from build123d import *

# Parameters (mm, degrees)
PAD_DEPTH    = 51.96
PAD001_DEPTH = 26
SKETCH002_R  = 2
POCKET_DEPTH = 45.899584
FILLET_R     = 3


with BuildPart() as part:
    # Sketch → Pad (new body)
    with BuildSketch(Plane.XY):
        with BuildLine():
            Line((-48.25, -23), (-52.123371, -6.118146))
            ThreePointArc((-47.25, 0), (-51.160929, -1.884774), (-52.123371, -6.118146))
            Line((-47.25, 0), (47.25, 0))
            ThreePointArc((52.123371, -6.118146), (51.160929, -1.884774), (47.25, 0))
            Line((52.123371, -6.118146), (48.25, -23))
            Line((48.25, -23), (47.25, -23))
            Line((47.25, -23), (47.25, -8))
            ThreePointArc((47.25, -8), (45.785534, -4.464466), (42.25, -3))
            Line((42.25, -3), (-42.25, -3))
            ThreePointArc((-42.25, -3), (-45.785534, -4.464466), (-47.25, -8))
            Line((-47.25, -8), (-47.25, -23))
            Line((-47.25, -23), (-48.25, -23))
        make_face()
    extrude(amount=PAD_DEPTH)

    # Sketch001 → Pad001 (join, symmetric)
    with BuildSketch(Plane.YZ):
        Polygon((0, 51.96), (29.99912, 51.96), (0, 0), (0, 6), (24.802968, 48.96), (0, 48.96), align=None)
    extrude(amount=PAD001_DEPTH, both=True)

    # Sketch002 (on Face15 of Pad001) → Pocket (cut, through all)
    with BuildSketch(Plane(origin=(0, 0, 0), x_dir=(-1, 0, 0), z_dir=(0, 0.866025, -0.5))):
        with Locations((-18, 49.99824)):
            Circle(SKETCH002_R)
        with Locations((18, 49.99824)):
            Circle(SKETCH002_R)
        with Locations((-18, 27.99824)):
            Circle(SKETCH002_R)
        with Locations((18, 27.99824)):
            Circle(SKETCH002_R)
    extrude(amount=-POCKET_DEPTH, mode=Mode.SUBTRACT)

    # Fillet
    fillet_edges = [part.edges().sort_by_distance(p)[0] for p in [
        (0, 0, 48.96),
        (0, 0, 6),
    ]]
    fillet(fillet_edges, radius=FILLET_R)


solid = part.part
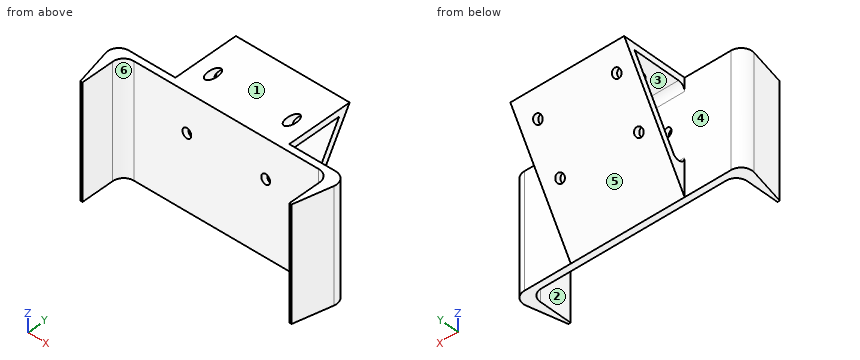
Check sheet for the modelled part. Datum: model origin and axes. Units: mm. Face numbers are marked on the shaded views. A direction names the side the tool comes from. Round coordinates to 2 decimals unless told otherwise and drop trailing zeros. Loops run counter-clockwise (first coordinate to the right, second up) from the corner with the lowest first, then second, coordinate; pieces in that order, holes last. Notation, with made-up numbers: (54, -23.5) - (69, -23.5) arc R26 cw to (69, -8.5) - close; hole circle Ø7 at (1, 10.5). An arc over 180 degrees is marked (long way). Answer as CSV lines item,"result". Start each with the question number.
Item 1: Scan lines: line 1 (Y direction, x = 37, z = 17); line 2 (X direction, y = -10, z = 9); line 3 (X direction, y = 0.5, z = 14.5). Record each from-to range of solid material in increasing order. Write a range as [from, to].
Item 2: Depth check by flat-ended pin: P1, Ø24, axis at y = 14.5, z = 34, coming from the +X side; P2, Ø11, axis at x = 8.5, y = 16.5, coming from the -Z side; P3, Ø12, axis at x = -36, z = 30, coming from the -Y side. Enter the tip coordinate at first touch or a pass-through.
Item 3: Section check B-B (y = -18). Record the boundary of the cut face in (x, z).
Item 4: Release check for a two-part mould opening along Z. For the marked faces 1, 2 and 3 record: +Z half, -Z half, draft (parallel to the pull), parting line (faces both ways), or undercut.
Item 5: Section check A-A (x = -9). Record the boundary of the cut face in (y, z).
Item 6: Set-up check for the marked faces 4, 5 and 6: record each of +Z, -Z, +X, -X, +Y, -Y from which the full face is reachable in a straight line by a thin tool's end or side.
Item 7: Section check C-C (z = 37.5). Record the boundary of the cut face in (x, y), and give its area (3 significant figures).
Item 8: Section check D-D (x = -37). Record the boundary of the cut face in (y, z), and give its area (3 significant figures).
Report:
1,line 1,"y = [-3, 0]"
1,line 2,"x = [-51.23, -47.25], [47.25, 51.23]"
1,line 3,"x = [-26, 26]"
2,P1,"stops at x = 26"
2,P2,"stops at z = 19.05"
2,P3,"stops at y = -3"
3,outline,"(-49.4, 0) - (-47.25, 0) - (-47.25, 51.96) - (-49.4, 51.96) - close; (47.25, 0) - (49.4, 0) - (49.4, 51.96) - (47.25, 51.96) - close"
4,face 1,"+Z half"
4,face 2,"draft"
4,face 3,"undercut"
5,outline,"(-3, 0) - (0, 0) - (30, 51.96) - (-3, 51.96) - close; hole (0, 17.2) arc R3 ccw to (5.6, 15.7) - (24.8, 48.96) - (3, 48.96) arc R3 ccw to (0, 45.96) - close"
6,face 4,"none"
6,face 5,"-Z, +X, -X, +Y"
6,face 6,"+Z, -Z, -Y"
7,outline,"(-52.12, -6.12) - (-48.25, -23) - (-47.25, -23) - (-47.25, -8) arc R5 cw to (-42.25, -3) - (42.25, -3) arc R5 cw to (47.25, -8) - (47.25, -23) - (48.25, -23) - (52.12, -6.12) arc R5 ccw to (47.25, 0) - (-47.25, 0) arc R5 ccw to start; (-26, 18.19) - (26, 18.19) - (26, 21.65) - (-26, 21.65) - close"
7,area,"624 mm2"
8,outline,"(-3, 0) - (0, 0) - (0, 51.96) - (-3, 51.96) - close"
8,area,"156 mm2"
